Geometry: see drawing. Coordinates: mm, zero at the bounding-box minimum. A direction names the side the tool comes from. Round coordinates to 2 decimals unless told otherwise and drop trailing zeros. Order: outer loops, then holes, each group sorted by start corner. A loop starts at its lowest first (then second) coordinate and runs counter-clockwise, first axis right, second up.
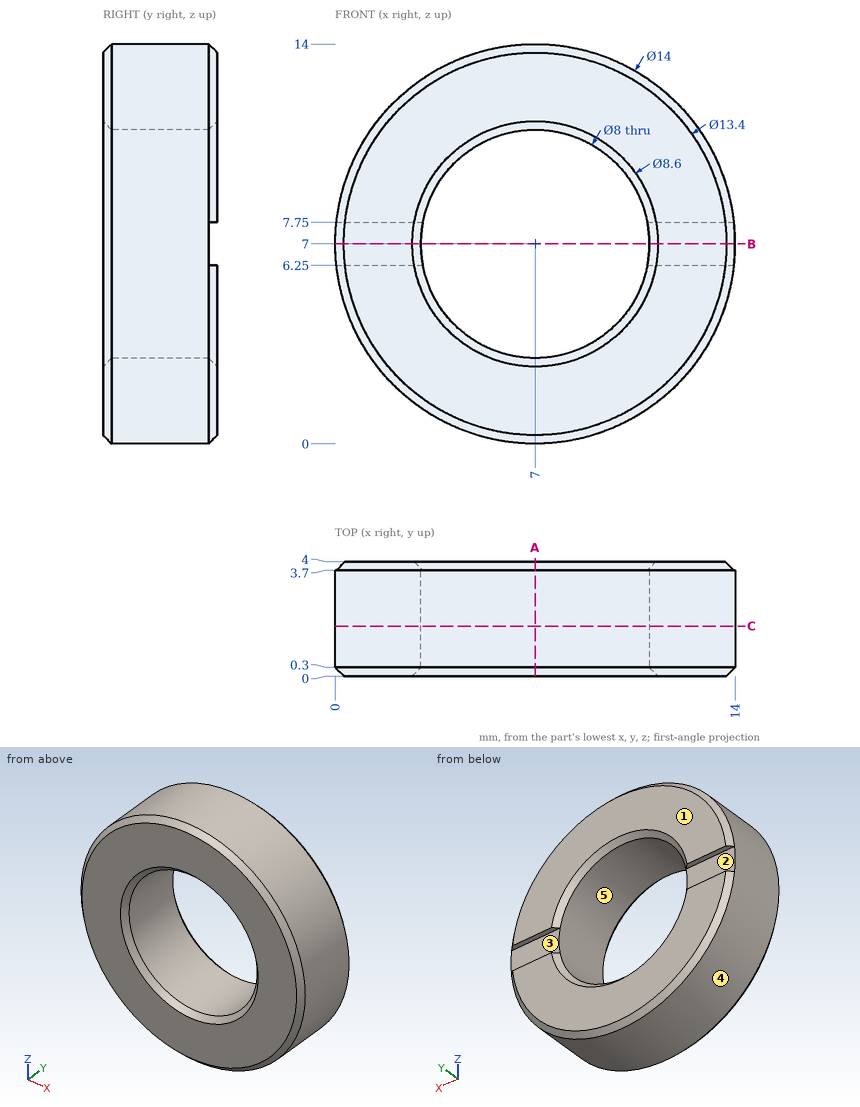
1. Section B-B on z = 7. Return loops of the section in (x, y).
2. Access query for the marked faces 1 and 2. Directions: +Z, -Z, +X, -X, +Y, -Y. A direction counts if a zero-diameter tool reaches every point of the face in a straight line with its end or side. Return the directions, or none.
3. Line query: line 1 along Z through (x, y) = (7, 1.7); line 2 along Z through (x, y) = (6.25, 2.2); line 3 along X through (y, z) = (3.5, 3.5). Output: solid intervals per line, ascending.
4. Pull-direction query (X, two-part tool) for the marked faces 3, 4 and 5; classes: released by +X, released by -X, zero draft, split by the parting line, or undercut.
5. Section C-C on y = 1.75. Return loops of the section in (x, z), plus the area to 3 significant figures.
6. First-contact query: pin 1 (1.5 mm diameter, centred on x = 10, z = 3.5, fed in from -Y); pin 2 (1 mm diameter, centred on y = 2, z = 5, fed in from -X). Flat tips, straight axial feed; report the tip coordinate or a pass-through.
7. Section A-A on x = 7. Return loops of the section in (y, z), plus the area to 3 significant figures.
Result:
1. outline: (0, 0.3) - (0.3, 0) - (2.7, 0) - (3, 0.3) - (3, 3.7) - (0, 3.7) - close; (11, 0.3) - (11.3, 0) - (13.7, 0) - (14, 0.3) - (14, 3.7) - (11, 3.7) - close
2. face 1: +Z, -Z, +X, -X, +Y
2. face 2: +X, -X, +Y
3. line 1: z = 0 to 3, 11 to 14
3. line 2: z = 0.04 to 3.07, 10.93 to 13.96
3. line 3: x = 0.94 to 5.06, 8.94 to 13.06
4. face 3: zero draft
4. face 4: split by the parting line
4. face 5: undercut
5. outline: circle Ø14 at (7, 7); hole circle Ø8 at (7, 7)
5. area: 104 mm2
6. pin 1: stops at y = 0
6. pin 2: stops at x = 0.16
7. outline: (0, 0.3) - (0.3, 0) - (3.7, 0) - (4, 0.3) - (4, 2.7) - (3.7, 3) - (0.3, 3) - (0, 2.7) - close; (0, 11.3) - (0.3, 11) - (3.7, 11) - (4, 11.3) - (4, 13.7) - (3.7, 14) - (0.3, 14) - (0, 13.7) - close
7. area: 23.6 mm2
